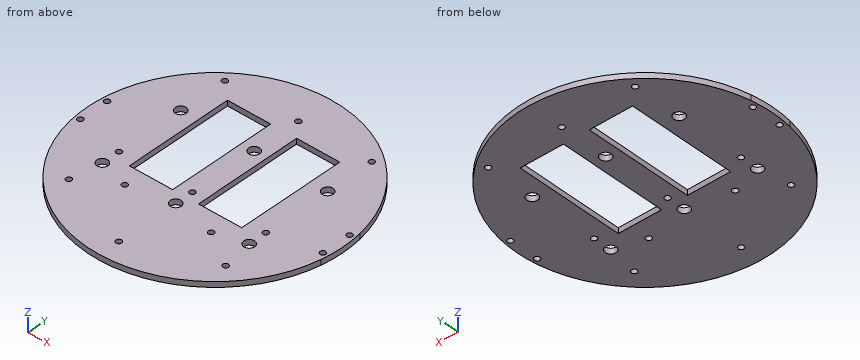
```python
from build123d import *

# Parameters (mm, degrees)
SKETCH1_R           = 1.651
BOSS_EXTRUDE2_DEPTH = 3.175
SKETCH5_W           = 36.105919561
SKETCH5_H           = 30.801250688
SKETCH5_W_2         = 35.958513686
SKETCH5_H_2         = 33.469345806
BOSS_EXTRUDE4_DEPTH = 3.175
SKETCH11_R          = 1.651
CUT_EXTRUDE7_DEPTH  = 4.175
BOSS_EXTRUDE6_DEPTH = 3.175
SKETCH13_R          = 3.175
CUT_EXTRUDE8_DEPTH  = 21.59
SKETCH14_W          = 25.4
SKETCH14_H          = 63.5
CUT_EXTRUDE9_DEPTH  = 46.482
SKETCH15_R          = 1.651
CUT_EXTRUDE10_DEPTH = 150.876


with BuildPart() as part:
    # Sketch1 → Boss-Extrude2 (new body)
    with BuildSketch(Plane.XY):
        with BuildLine():
            Line((-73.845886141, 12.7), (-56.065886141, 12.7))
            Line((-56.065886141, 12.7), (-56.065886141, -12.7))
            Line((-56.065886141, -12.7), (-73.845886141, -12.7))
            ThreePointArc((-73.845886141, -12.7), (0, -74.93), (73.845886141, -12.7))
            Line((73.845886141, -12.7), (56.065886141, -12.7))
            Line((56.065886141, -12.7), (56.065886141, 12.7))
            Line((56.065886141, 12.7), (73.845886141, 12.7))
            ThreePointArc((73.845886141, 12.7), (0, 74.93), (-73.845886141, 12.7))
        make_face()
        with Locations((-45.466, 11.049)):
            Circle(SKETCH1_R, mode=Mode.SUBTRACT)
        with Locations((-20.067270032, 10.795)):
            Circle(SKETCH1_R, mode=Mode.SUBTRACT)
        with Locations((-20.067270032, -10.795)):
            Circle(SKETCH1_R, mode=Mode.SUBTRACT)
        with Locations((-45.466, -11.049)):
            Circle(SKETCH1_R, mode=Mode.SUBTRACT)
        with Locations((45.466, -11.049)):
            Circle(SKETCH1_R, mode=Mode.SUBTRACT)
        with Locations((20.067270032, -10.795)):
            Circle(SKETCH1_R, mode=Mode.SUBTRACT)
        with Locations((20.067270032, 10.795)):
            Circle(SKETCH1_R, mode=Mode.SUBTRACT)
        with Locations((45.466, 11.049)):
            Circle(SKETCH1_R, mode=Mode.SUBTRACT)
    extrude(amount=BOSS_EXTRUDE2_DEPTH)

    # Sketch5 → Boss-Extrude4 (add)
    with BuildSketch(Plane(origin=(0, 0, 0), x_dir=(-1, 0, 0), z_dir=(0, 0, -1))):
        with Locations((34.78484389, -0.38515144)):
            Rectangle(SKETCH5_W, SKETCH5_H)
        with Locations((-32.830563904, 0.948896119)):
            Rectangle(SKETCH5_W_2, SKETCH5_H_2)
    extrude(amount=-BOSS_EXTRUDE4_DEPTH)

    # Sketch11 → Cut-Extrude7 (cut, through all)
    with BuildSketch(Plane(origin=(0, 0, 0), x_dir=(-1, 0, 0), z_dir=(0, 0, -1))):
        with Locations((43.18, 53.975)):
            Circle(SKETCH11_R)
        with Locations((0, 53.975)):
            Circle(SKETCH11_R)
        with Locations((0, -14.605)):
            Circle(SKETCH11_R)
        with Locations((43.18, -14.605)):
            Circle(SKETCH11_R)
        with Locations((-43.18, 53.975)):
            Circle(SKETCH11_R)
        with Locations((-43.18, -14.605)):
            Circle(SKETCH11_R)
        with Locations((-25.4, -30.48)):
            Circle(SKETCH11_R)
        with Locations((-46.101, -43.8609994)):
            Circle(SKETCH11_R)
        with Locations((46.101, -43.8609994)):
            Circle(SKETCH11_R)
        with Locations((0, -62.3219988)):
            Circle(SKETCH11_R)
        with Locations((25.4, -30.48)):
            Circle(SKETCH11_R)
    extrude(amount=-CUT_EXTRUDE7_DEPTH, mode=Mode.SUBTRACT)

    # Sketch12 → Boss-Extrude6 (add)
    with BuildSketch(Plane(origin=(0, 0, 0), x_dir=(-1, 0, 0), z_dir=(0, 0, -1))):
        with BuildLine():
            Line((-54.995250635, 50.892310889), (-54.566459663, -51.351790425))
            ThreePointArc((-54.566459663, -51.351790425), (-74.929341077, -0.314238422), (-54.995250635, 50.892310889))
        make_face()
        with BuildLine():
            Line((54.995250635, 50.892310889), (54.995250635, -50.892310889))
            ThreePointArc((54.995250635, -50.892310889), (74.93, 0), (54.995250635, 50.892310889))
        make_face()
    extrude(amount=-BOSS_EXTRUDE6_DEPTH)

    # Sketch13 → Cut-Extrude8 (cut)
    with BuildSketch(Plane(origin=(0, 0, 0), x_dir=(-1, 0, 0), z_dir=(0, 0, -1))):
        with Locations((0, 25.4)):
            Circle(SKETCH13_R)
        with Locations((43.18, 25.4)):
            Circle(SKETCH13_R)
        with Locations((-43.18, 25.4)):
            Circle(SKETCH13_R)
        with Locations((-43.18, -25.4)):
            Circle(SKETCH13_R)
        with Locations((0, -25.4)):
            Circle(SKETCH13_R)
        with Locations((43.18, -25.4)):
            Circle(SKETCH13_R)
    extrude(amount=-CUT_EXTRUDE8_DEPTH, mode=Mode.SUBTRACT)

    # Sketch14 → Cut-Extrude9 (cut)
    with BuildSketch(Plane(origin=(0, 0, 0), x_dir=(-1, 0, 0), z_dir=(0, 0, -1))):
        with Locations((-20.32, 12.7)):
            Rectangle(SKETCH14_W, SKETCH14_H)
        with Locations((20.32, 12.7)):
            Rectangle(SKETCH14_W, SKETCH14_H)
    extrude(amount=-CUT_EXTRUDE9_DEPTH, mode=Mode.SUBTRACT)

    # Sketch15 → Cut-Extrude10 (cut)
    with BuildSketch(Plane(origin=(-30.092005081, 4.08352975, -73.025), x_dir=(-1, 0, 0), z_dir=(0, 0, -1))):
        with Locations((-101.395980802, -12.71952975)):
            Circle(SKETCH15_R)
        with Locations((-101.395980802, 4.55247025)):
            Circle(SKETCH15_R)
        with Locations((41.211970641, -12.71952975)):
            Circle(SKETCH15_R)
        with Locations((41.211970641, 4.55247025)):
            Circle(SKETCH15_R)
    extrude(amount=-CUT_EXTRUDE10_DEPTH, mode=Mode.SUBTRACT)


solid = part.part
```
Geometry: final body of the model. Coordinates: model frame, mm. Round coordinates to 2 decimals unless told otherwise and drop trailing zeros. Order: outer loops, then holes, each group sorted by start corner. A loop starts at its lowest first (then second) coordinate and runs counter-clockwise, first axis right, second up. Notation, with made-up numbers: (50.5, 65) - (60.5, 65) arc R9 ccw to (60.5, 74) - close; hole circle Ø10 at (58.25, 33). An arc over 180 degrees is marked (long way). Write item = value, one per line. Start each with the question number.
Q1. Cut plane C-C on y = -25.4. Return the cut outline in (x, z) (3 decimals).
Q2. Pin query (flat end, axial travel): pin 1 (2.5 mm diameter, centred on x = -43.18, y = 53.975, fed in from -Z); pin 2 (1.5 mm diameter, centred on x = 32, z = 1, fed in from -Y); pin 3 (1 mm diameter, centred on x = 21, z = 1, fed in from -Y); pin 4 (1.6 mm diameter, centred on x = -18.5, z = 1.5, fed in from +Y). Return the tip coordinate at first contact, or that it passes through.
Q3. Ray query, line 1 (Y direction, x = -25.4, z = 2.5); line 2 (X direction, y = 40, z = 1.55); line 3 (Y direction, x = -43.18, z = 1.6) (3 decimals). Return the intervals inside material, ascending. Write a range as from..to.
Q4. Cut plane B-B on y = 25.4. Return the cut outline in (x, z) (3 decimals).
Q5. Cut plane D-D on x = 54. Return the cut outline in (y, z) (3 decimals).
Q6. Cut plane A-A on z = 2.55. Give the number of separate pieces and of enclosed holes in the cut face, and give its area (3 significant figures).
Outcome:
q1.outline = (-70.494, 0) - (-46.355, 0) - (-46.355, 3.175) - (-70.494, 3.175) - close; (-40.005, 0) - (-3.175, 0) - (-3.175, 3.175) - (-40.005, 3.175) - close; (3.175, 0) - (40.005, 0) - (40.005, 3.175) - (3.175, 3.175) - close; (46.355, 0) - (70.494, 0) - (70.494, 3.175) - (46.355, 3.175) - close
q2.pin_1 = through
q2.pin_2 = -68.1
q2.pin_3 = -72.07
q2.pin_4 = 72.81
q3.line_1 = -70.49..-32.13, -28.83..-19.05, 44.45..70.49
q3.line_2 = -63.36..-33.02, -7.62..7.62, 33.02..63.36
q3.line_3 = -61.237..-28.575, -22.225..-16.256, -12.954..22.225, 28.575..52.324, 55.626..61.237
q4.outline = (-70.494, 0) - (-46.355, 0) - (-46.355, 3.175) - (-70.494, 3.175) - close; (-40.005, 0) - (-33.02, 0) - (-33.02, 3.175) - (-40.005, 3.175) - close; (-7.62, 0) - (-3.175, 0) - (-3.175, 3.175) - (-7.62, 3.175) - close; (3.175, 0) - (7.62, 0) - (7.62, 3.175) - (3.175, 3.175) - close; (33.02, 0) - (40.005, 0) - (40.005, 3.175) - (33.02, 3.175) - close; (46.355, 0) - (70.494, 0) - (70.494, 3.175) - (46.355, 3.175) - close
q5.outline = (-51.947, 0) - (51.947, 0) - (51.947, 3.175) - (-51.947, 3.175) - close
q6.separate_pieces = 1
q6.enclosed_holes = 23
q6.area = 14,100 mm^2
